Model file for the job. Use its own axes, mm. Round coordinates to 2 decimals unless told otherwise and drop trailing zeros. Loops run counter-clockwise (first coordinate to the right, second up) from the corner with the lowest first, then second, coordinate; pieces in that order, holes last. Notation, with made-up numbers: (-7, 35.5) - (31, 35.5) arc R17 cw to (31, 54.5) - close; hole circle Ø1 at (-3, 61). An arc over 180 degrees is marked (long way). Answer as a JSON object with one key per item and string values.
from build123d import *

# Parameters (mm, degrees)
SKETCH1_W           = 7
SKETCH1_H           = 7
BOSS_EXTRUDE1_DEPTH = 1
SKETCH2_W           = 0.3
SKETCH2_H           = 0.25
BOSS_EXTRUDE2_DEPTH = 0.3
SKETCH3_W           = 0.3
SKETCH3_H           = 0.25
BOSS_EXTRUDE3_DEPTH = 0.3
SKETCH4_W           = 0.3
SKETCH4_H           = 0.25
BOSS_EXTRUDE4_DEPTH = 0.3
SKETCH5_W           = 0.3
SKETCH5_H           = 0.25
BOSS_EXTRUDE5_DEPTH = 0.3


with BuildPart() as part:
    # Sketch1 → Boss-Extrude1 (new body)
    with BuildSketch(Plane(origin=(0, 0, 0), x_dir=(1, 0, 0), z_dir=(0, 1, 0))):
        with Locations((3.5, 3.5)):
            Rectangle(SKETCH1_W, SKETCH1_H)
    extrude(amount=BOSS_EXTRUDE1_DEPTH)

    # Sketch2 → Boss-Extrude2 (add)
    with BuildSketch(Plane.XY):
        with Locations((0.65, 0.125)):
            Rectangle(SKETCH2_W, SKETCH2_H)
        with Locations((1.22, 0.125)):
            Rectangle(SKETCH2_W, SKETCH2_H)
        with Locations((1.79, 0.125)):
            Rectangle(SKETCH2_W, SKETCH2_H)
        with Locations((2.36, 0.125)):
            Rectangle(SKETCH2_W, SKETCH2_H)
        with Locations((2.93, 0.125)):
            Rectangle(SKETCH2_W, SKETCH2_H)
        with Locations((3.5, 0.125)):
            Rectangle(SKETCH2_W, SKETCH2_H)
        with Locations((4.07, 0.125)):
            Rectangle(SKETCH2_W, SKETCH2_H)
        with Locations((4.64, 0.125)):
            Rectangle(SKETCH2_W, SKETCH2_H)
        with Locations((5.21, 0.125)):
            Rectangle(SKETCH2_W, SKETCH2_H)
        with Locations((5.78, 0.125)):
            Rectangle(SKETCH2_W, SKETCH2_H)
        with Locations((6.35, 0.125)):
            Rectangle(SKETCH2_W, SKETCH2_H)
    extrude(amount=BOSS_EXTRUDE2_DEPTH)

    # Sketch3 → Boss-Extrude3 (add)
    with BuildSketch(Plane(origin=(7, 0, 0), x_dir=(0, 0, -1), z_dir=(1, 0, 0))):
        with Locations((0.65, 0.125)):
            Rectangle(SKETCH3_W, SKETCH3_H)
        with Locations((1.22, 0.125)):
            Rectangle(SKETCH3_W, SKETCH3_H)
        with Locations((1.79, 0.125)):
            Rectangle(SKETCH3_W, SKETCH3_H)
        with Locations((2.36, 0.125)):
            Rectangle(SKETCH3_W, SKETCH3_H)
        with Locations((2.93, 0.125)):
            Rectangle(SKETCH3_W, SKETCH3_H)
        with Locations((3.5, 0.125)):
            Rectangle(SKETCH3_W, SKETCH3_H)
        with Locations((4.07, 0.125)):
            Rectangle(SKETCH3_W, SKETCH3_H)
        with Locations((4.64, 0.125)):
            Rectangle(SKETCH3_W, SKETCH3_H)
        with Locations((5.21, 0.125)):
            Rectangle(SKETCH3_W, SKETCH3_H)
        with Locations((5.78, 0.125)):
            Rectangle(SKETCH3_W, SKETCH3_H)
        with Locations((6.35, 0.125)):
            Rectangle(SKETCH3_W, SKETCH3_H)
    extrude(amount=BOSS_EXTRUDE3_DEPTH)

    # Sketch4 → Boss-Extrude4 (add)
    with BuildSketch(Plane(origin=(0, 0, -7), x_dir=(-1, 0, 0), z_dir=(0, 0, -1))):
        with Locations((-6.35, 0.125)):
            Rectangle(SKETCH4_W, SKETCH4_H)
        with Locations((-5.78, 0.125)):
            Rectangle(SKETCH4_W, SKETCH4_H)
        with Locations((-5.21, 0.125)):
            Rectangle(SKETCH4_W, SKETCH4_H)
        with Locations((-4.64, 0.125)):
            Rectangle(SKETCH4_W, SKETCH4_H)
        with Locations((-4.07, 0.125)):
            Rectangle(SKETCH4_W, SKETCH4_H)
        with Locations((-3.5, 0.125)):
            Rectangle(SKETCH4_W, SKETCH4_H)
        with Locations((-2.93, 0.125)):
            Rectangle(SKETCH4_W, SKETCH4_H)
        with Locations((-2.36, 0.125)):
            Rectangle(SKETCH4_W, SKETCH4_H)
        with Locations((-1.79, 0.125)):
            Rectangle(SKETCH4_W, SKETCH4_H)
        with Locations((-1.22, 0.125)):
            Rectangle(SKETCH4_W, SKETCH4_H)
        with Locations((-0.65, 0.125)):
            Rectangle(SKETCH4_W, SKETCH4_H)
    extrude(amount=BOSS_EXTRUDE4_DEPTH)

    # Sketch5 → Boss-Extrude5 (add)
    with BuildSketch(Plane.ZY):
        with Locations((-6.35, 0.125)):
            Rectangle(SKETCH5_W, SKETCH5_H)
        with Locations((-5.78, 0.125)):
            Rectangle(SKETCH5_W, SKETCH5_H)
        with Locations((-5.21, 0.125)):
            Rectangle(SKETCH5_W, SKETCH5_H)
        with Locations((-4.64, 0.125)):
            Rectangle(SKETCH5_W, SKETCH5_H)
        with Locations((-4.07, 0.125)):
            Rectangle(SKETCH5_W, SKETCH5_H)
        with Locations((-3.5, 0.125)):
            Rectangle(SKETCH5_W, SKETCH5_H)
        with Locations((-2.93, 0.125)):
            Rectangle(SKETCH5_W, SKETCH5_H)
        with Locations((-2.36, 0.125)):
            Rectangle(SKETCH5_W, SKETCH5_H)
        with Locations((-1.79, 0.125)):
            Rectangle(SKETCH5_W, SKETCH5_H)
        with Locations((-1.22, 0.125)):
            Rectangle(SKETCH5_W, SKETCH5_H)
        with Locations((-0.65, 0.125)):
            Rectangle(SKETCH5_W, SKETCH5_H)
    extrude(amount=BOSS_EXTRUDE5_DEPTH)


solid = part.part
1) Slice it at B-B on x = 1.25. List the corners of the cut face in (y, z), then the cut area to 3 significant figures.
Values follow:
{"outline": "(0, -7.3) - (0.25, -7.3) - (0.25, -7) - (1, -7) - (1, 0) - (0.25, 0) - (0.25, 0.3) - (0, 0.3) - close", "area": "7.15 mm²"}
2) Probe probe 1 along X at (y, z) = (0.3, -4.5); probe 2 along Z at (x, y) = (3.75, 0.5); probe 3 along Y at (x, z) = (7.25, -4.75). List the from-to ranges inside material, lowest first.
Values follow:
{"probe 1": "0 to 7", "probe 2": "-7 to 0", "probe 3": "0 to 0.25"}
3) Slice it at C-C on y = 0.5. List the corners of the cut face in (x, z), then the cut area to 3 significant figures.
Values follow:
{"outline": "(0, -7) - (7, -7) - (7, 0) - (0, 0) - close", "area": "49.0 mm²"}
4) Slice it at D-D on z = -3.75. List the corners of the cut face in (x, y).
Values follow:
{"outline": "(0, 0) - (7, 0) - (7, 1) - (0, 1) - close"}
5) Drop a flat-ended pin along its axis: P1, Ø1, axis at x = 5.5, z = -4.5, coming from the -Y side. Give the stop position or say it passes through.
Values follow:
{"P1": "y = 0"}
6) Slice it at A-A on z = -1.75. List the corners of the cut face in (x, y), then the cut area to 3 significant figures.
Values follow:
{"outline": "(-0.3, 0) - (7.3, 0) - (7.3, 0.25) - (7, 0.25) - (7, 1) - (0, 1) - (0, 0.25) - (-0.3, 0.25) - close", "area": "7.15 mm²"}
